Read the model definition and answer for the solid it produces. Units are mm, in the model's axes. A direction names the side the tool comes from. Coordinates: 2 decimals unless noted, no trailing zeros. Loops run counter-clockwise (first coordinate to the right, second up) from the corner with the lowest first, then second, coordinate; pieces in that order, holes last.
from build123d import *

# Parameters (mm, degrees)
F0_W     = 6.35
F0_H     = 6.35
F1_DEPTH = 19.05
F2_R     = 4.826
F3_DEPTH = 93.9810005078


# Not quite as in the source:
# - ends of sketch curves that miss each other by under 0.0002 mm in the source are joined


with BuildPart() as f1:
    # F0 (on Front) → F1 (new body)
    with BuildSketch(Plane.XZ):
        with BuildLine():
            Line((-40.64, -63.5), (-40.64, 0))
            ThreePointArc((-40.64, 0), (-34.1462652747, 22.0372903913), (-16.7402870182, 37.0320454545))
            ThreePointArc((-16.7402870182, 37.0320454545), (-9.7390716727, 44.3123236883), (0, 46.99))
            ThreePointArc((0, 46.99), (-33.2269478275, 33.2269478275), (-46.9900002539, 0))
            Line((-46.9900002539, 0), (-46.9900002539, -63.5))
            Line((-46.9900002539, -63.5), (-40.64, -63.5))
        make_face()
        with BuildLine():
            ThreePointArc((0, 46.99), (-9.7390716727, 44.3123236883), (-16.7402870182, 37.0320454545))
            ThreePointArc((-16.7402870182, 37.0320454545), (-8.5623382423, 39.727773205), (2.25e-08, 40.64))
            ThreePointArc((2.25e-08, 40.64), (8.5623382643, 39.7277732002), (16.7402870182, 37.0320454545))
            ThreePointArc((16.7402870182, 37.0320454545), (9.7390716727, 44.3123236883), (0, 46.99))
        make_face()
        with BuildLine():
            ThreePointArc((16.7402870182, 37.0320454545), (34.1462652747, 22.0372903913), (40.64, 0))
            Line((40.64, 0), (40.64, -63.5))
            Line((40.64, -63.5), (46.9900002539, -63.5))
            Line((46.9900002539, -63.5), (46.9900002539, 0))
            ThreePointArc((46.9900002539, 0), (33.2269478275, 33.2269478275), (0, 46.9900002539))
            ThreePointArc((0, 46.9900002539), (9.7390716727, 44.3123236883), (16.7402870182, 37.0320454545))
        make_face()
        with BuildLine():
            ThreePointArc((19.05, 27.94), (18.463544726, 32.6304174816), (16.7402870182, 37.0320454545))
            ThreePointArc((16.7402870182, 37.0320454545), (8.5623382643, 39.7277732002), (2.25e-08, 40.64))
            ThreePointArc((2.25e-08, 40.64), (8.980256129, 36.9202561131), (12.7, 27.94))
            Line((12.7, 27.94), (19.05, 27.94))
        make_face()
        with BuildLine():
            ThreePointArc((2.25e-08, 40.64), (-8.5623382423, 39.727773205), (-16.7402870182, 37.0320454545))
            ThreePointArc((-16.7402870182, 37.0320454545), (-18.463544726, 32.6304174816), (-19.05, 27.94))
            Line((-19.05, 27.94), (-12.7, 27.94))
            ThreePointArc((-12.7, 27.94), (-8.9802561131, 36.920256129), (2.25e-08, 40.64))
        make_face()
        with Locations((15.875, 24.765)):
            Rectangle(F0_W, F0_H)
        with Locations((-15.875, 24.765)):
            Rectangle(F0_W, F0_H)
    extrude(amount=-F1_DEPTH)

    # F2 (on face) → F3 (cut, through all)
    with BuildSketch(Plane.YZ.offset(46.9900002539)):
        with Locations((9.525, -50.8)):
            Circle(F2_R)
    extrude(amount=-F3_DEPTH, mode=Mode.SUBTRACT)


solid = f1.part
Q1. Which of the six approach directions +Z, -Z, +X, -X, +Y, -Y give full straight-line access (tool end or side, diameter ignored) to faces 1 (the face through (-12.7, 9, 25)), 2 (the face through (44, 9, -63.5))?
Findings below:
face 1: -Z, +Y, -Y
face 2: -Z, +X, -X, +Y, -Y
Q2. A cutting plane is placed at B-B (y = 6.5). Give the vertices of the cut face in (x, z).
Findings below:
outline: (-46.99, -63.5) - (-40.64, -63.5) - (-40.64, -54.56) - (-46.99, -54.56) - close; (-46.99, -47.04) - (-40.64, -47.04) - (-40.64, 0) arc R40.64 cw to (-16.74, 37.03) arc R19.05 ccw to (-19.05, 27.94) - (-19.05, 21.59) - (-12.7, 21.59) - (-12.7, 27.94) arc R12.7 cw to (12.7, 27.94) - (12.7, 21.59) - (19.05, 21.59) - (19.05, 27.94) arc R19.05 ccw to (16.74, 37.03) arc R40.64 cw to (40.64, 0) - (40.64, -47.04) - (46.99, -47.04) - (46.99, 0) arc R46.99 ccw to (-46.99, 0) - close; (40.64, -63.5) - (46.99, -63.5) - (46.99, -54.56) - (40.64, -54.56) - close
Q3. A cutting plane is placed at C-C (z = -50.8). Give the vertices of the cut face in (x, y).
Findings below:
outline: (-46.99, 0) - (-40.64, 0) - (-40.64, 4.7) - (-46.99, 4.7) - close; (-46.99, 14.35) - (-40.64, 14.35) - (-40.64, 19.05) - (-46.99, 19.05) - close; (40.64, 0) - (46.99, 0) - (46.99, 4.7) - (40.64, 4.7) - close; (40.64, 14.35) - (46.99, 14.35) - (46.99, 19.05) - (40.64, 19.05) - close
Q4. A cutting plane is placed at D-D (y = 12). Give the vertices of the cut face in (x, z).
Findings below:
outline: (-46.99, -63.5) - (-40.64, -63.5) - (-40.64, -54.94) - (-46.99, -54.94) - close; (-46.99, -46.66) - (-40.64, -46.66) - (-40.64, 0) arc R40.64 cw to (-16.74, 37.03) arc R19.05 ccw to (-19.05, 27.94) - (-19.05, 21.59) - (-12.7, 21.59) - (-12.7, 27.94) arc R12.7 cw to (12.7, 27.94) - (12.7, 21.59) - (19.05, 21.59) - (19.05, 27.94) arc R19.05 ccw to (16.74, 37.03) arc R40.64 cw to (40.64, 0) - (40.64, -46.66) - (46.99, -46.66) - (46.99, 0) arc R46.99 ccw to (-46.99, 0) - close; (40.64, -63.5) - (46.99, -63.5) - (46.99, -54.94) - (40.64, -54.94) - close
Q5. Determine the mould class of faces 3 (the face through (-43.77, 8.48, -55.51)), 4 (the face through (-14, 0, 25)), 5 (the face through (-40.64, 9, -32)) for opening direction Y: +Y half, -Y half, draft (parallel to the pull), parting line (faces both ways), or undercut.
Findings below:
face 3: undercut
face 4: -Y half
face 5: draft
Q6. Flat-ended cylindrical pins translate along their axes: pin 1 Ø1 at (x, y) = (14.5, 9) entering from -Z; pin 2 Ø1.9 at (y, z) = (6.5, 24) entering from +X; pin 3 Ø7 at (y, z) = (12, 25) entering from +X. Find the tip coordinate at first contact, or state that the pin passes through.
Findings below:
pin 1: stops at z = 21.59
pin 2: stops at x = 40.95
pin 3: stops at x = 41.78
Q7. Straight lines are drawn through the part: probe 1 along X at (y, z) = (12.75, -15); probe 2 along X at (y, z) = (9.5, 27); probe 3 along X at (y, z) = (13.75, 20.5). For each, find the intervals that lie inside material, in ascending order.
Findings below:
probe 1: x = -46.99 to -40.64, 40.64 to 46.99
probe 2: x = -38.46 to -30.37, -19.05 to -12.7, 12.7 to 19.05, 30.37 to 38.46
probe 3: x = -42.28 to -35.09, 35.09 to 42.28
Q8. A cutting plane is placed at A-A (z = -24). Give the vertices of the cut face in (x, y), then the cut area to 3 significant figures.
Findings below:
outline: (-46.99, 0) - (-40.64, 0) - (-40.64, 19.05) - (-46.99, 19.05) - close; (40.64, 0) - (46.99, 0) - (46.99, 19.05) - (40.64, 19.05) - close
area: 242 mm2
